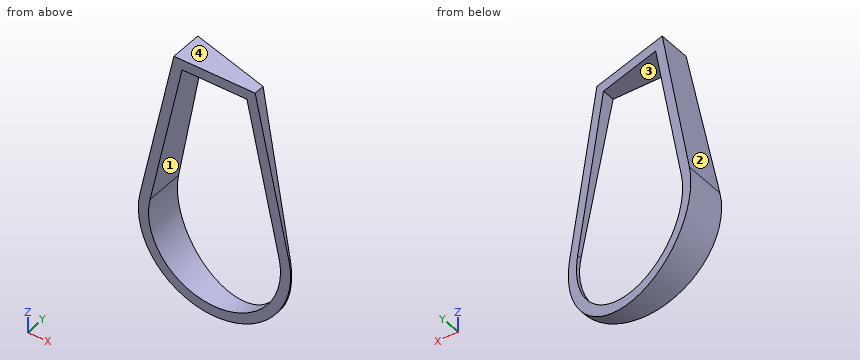
```python
from build123d import *

# Parameters (mm, degrees)
EXTRUDE_1_DEPTH     = 70
CUT_EXTRUDE_1_DEPTH = 266.612499706


with BuildPart() as part:
    # 草图1 → 凸台-拉伸1 (new body)
    with BuildSketch(Plane(origin=(0, 0, 0), x_dir=(1, 0, 0), z_dir=(0, 1, 0))):
        with BuildLine():
            Line((-73.31, -15.831737113), (-40.016432831, -170))
            Line((-40.016432831, -170), (40.016432831, -170))
            Line((40.016432831, -170), (73.31, -15.831737113))
            ThreePointArc((73.31, -15.831737113), (0, 75), (-73.31, -15.831737113))
        make_face()
        with BuildLine():
            Line((-63.535333333, -13.720838831), (-31.945465312, -160))
            Line((-31.945465312, -160), (31.945465312, -160))
            Line((31.945465312, -160), (63.535333333, -13.720838831))
            ThreePointArc((63.535333333, -13.720838831), (0, 65), (-63.535333333, -13.720838831))
        make_face(mode=Mode.SUBTRACT)
    extrude(amount=EXTRUDE_1_DEPTH)

    # 草图2 → 切除-拉伸1 (cut, through all)
    with BuildSketch(Plane.XY.offset(170)):
        Polygon((-80, 42.871870789), (80, 0), (80, 71.175543423), (-80, 71.175543423), align=None)
    extrude(amount=-CUT_EXTRUDE_1_DEPTH, mode=Mode.SUBTRACT)


solid = part.part
```
Read the model definition and answer for the solid it produces. Units are mm, in the model's axes. Face numbers are marked on the shaded views. A direction names the side the tool comes from. Give positions to 0.01 mm unless a question says otherwise; leave off trailing zeros. Order: outer loops, then holes, each group sorted by start corner. A loop starts at its lowest first (then second) coordinate and runs counter-clockwise, first axis right, second up.
(1) For a pull along Z with two mould halves and no side action, classify the marked faces 3 and 4 as released by +Z, released by -Z, zero draft, split by the parting line, or undercut.
(2) Find section B-B (x = 48.5). Give the vertices of the cut face in (y, z), plus the area to 3 significant figures.
(3) Find section D-D (y = 36). Give the vertices of the cut face in (x, z), plus the area to 3 significant figures.
(4) For the marked faces 1 and 2, determine the directions among +Z, -Z, +X, -X, +Y, -Y from which every point of the face is accessible in a straight line to the end or side of a thin tool.
(5) Straight lines are drawn through the part: L1, parallel to Z at x = 0, y = 17.5; L2, parallel to X at y = 27, z = 0; L3, parallel to X at y = 20, z = 2.5. For each, find the intervals that lie inside material, in ascending order.
(6) Given pin 1 (6 mm diameter, centred on y = 12, z = -33, fed in from -X); pin 2 (3 mm diameter, centred on y = 28.5, z = 34, fed in from +X); pin 3 (15 mm diameter, centred on x = 8, y = 18.5, fed in from -Z), each flat-ended and moving along its own axis, determine where each tip first touches the part or whether it passes through.
(7) Find section A-A (z = -43). Give the vertices of the cut face in (x, y), plus the area to 3 significant figures.
(8) Find section C-C (y = 22). Give the vertices of the cut face in (x, z).
Result sheet:
1. face 3: undercut
1. face 4: released by +Z
2. outline: (0, -57.21) - (8.44, -57.21) - (8.44, -43.28) - (0, -43.28) - close; (0, 83.34) - (8.44, 83.34) - (8.44, 130.72) - (0, 130.72) - close
2. area: 517 mm2
3. outline: (-73.31, 15.83) arc R75 ccw to (-54.35, -51.68) - (-54.35, -35.65) arc R65 cw to (-63.54, 13.72) - (-54.35, 56.24) - (-54.35, 103.61) - close
3. area: 1,290 mm2
4. face 1: +Y, -Y
4. face 2: +Z, -X, +Y, -Y
5. L1: z = -75 to -65, 160 to 170
5. L2: x = -75 to -65
5. L3: x = -74.96 to -64.95
6. pin 1: stops at x = -68.74
6. pin 2: stops at x = -58.83
6. pin 3: stops at z = -75
7. outline: (-61.45, 0) - (-48.74, 0) - (-48.74, 34.5) - (-61.45, 37.9) - close; (48.74, 0) - (61.45, 0) - (61.45, 4.97) - (48.74, 8.37) - close
7. area: 545 mm2
8. outline: (-73.31, 15.83) arc R75 ccw to (-2.11, -74.97) - (-2.11, -64.97) arc R65 cw to (-63.54, 13.72) - (-31.95, 160) - (-2.11, 160) - (-2.11, 170) - (-40.02, 170) - close
